Input: part model. Units: mm. Frame: model coordinates. A direction names the side the tool comes from. Coordinates: 2 decimals unless noted, no trailing zeros. Order: outer loops, then holes, each group sorted by start corner. A loop starts at its lowest first (then second) coordinate and runs counter-clockwise, first axis right, second up. Notation, with made-up numbers: (-39, 64) -> (-20, 64) arc R26 cw to (-20, 97) -> close; hole circle Ø4 at (7.5, 7.5). An arc over 180 degrees is marked (long way). Use one line per item in the form item = value. Start each with the question number.
1) Pin query (flat end, axial travel): pin 1 (4 mm diameter, centred on x = 17.5, y = -8, fed in from +Z); pin 2 (0.9 mm diameter, centred on x = 63, y = 21.5, fed in from +Z); pin 3 (1 mm diameter, centred on x = 22, y = 17.5, fed in from +Z); pin 4 (2.5 mm diameter, centred on x = 68.6, z = 64, fed in from +Y). Return the tip coordinate at first contact, or that it passes through.
2) Draft query along Z for faces 1 (the flat face through (-7.6, 16.25, 9.93)), 2 (the cylindrical face through (-11.53, 21.52, -17.5)), 3 (the cylindrical face through (28.83, 22.24, 65.004)). Return one class per face: pulls with the +Z half, pulls with the -Z half, needs draft (parallel to the pull), parting line crosses it, or undercut.
3) Section query C-C on z = 29. Output: boundary loops of the cut face in (x, y).
4) Ray query, line 1 along X through (y, z) = (21.65, 64); line 2 along Z through (x, y) = (68.6, 22.3); line 3 along X through (y, z) = (22, -16). Return the intervals inside material, ascending.
5) Access query for faces 4 (the flat face through (19, -7, 4)), 5 (the flat face through (18, -3.5, 3)), 6 (the flat face through (0, 22, -9)), 7 (the flat face through (64, 21, 74)). Directions: +Z, -Z, +X, -X, +Y, -Y. A direction counts if a zero-diameter tool reaches every point of the face in a straight line with its end or side. Return the directions, or none.
6) Section query A-A on z = -4. Output: boundary loops of the cut face in (x, y).
7) Section query B-B on y = -8. Count the separate pieces of the cut face and the enclosed holes in it, then the cut area to 3 significant figures.
from build123d import *

# Parameters (mm, degrees)
SKETCH_1_W               = 57
SKETCH_1_H               = 23
EXTRUDE_1_DEPTH          = 80
SKETCH_2_W               = 55
SKETCH_2_H               = 20
CUT_EXTRUDE_1_DEPTH      = 75
SKETCH_3_W               = 6
SKETCH_3_H               = 6
EXTRUDE_2_DEPTH          = 6
SKETCH_4_W               = 6
SKETCH_4_H               = 6.5
SKETCH_4_R               = 1.5
EXTRUDE_3_DEPTH          = 3
MIRROR_2_COPY_1_SKETCH_W = 6
MIRROR_2_COPY_1_SKETCH_H = 6.5
MIRROR_2_COPY_1_SKETCH_R = 1.5
MIRROR_2_COPY_1_DEPTH    = 3
CUT_EXTRUDE_3_DEPTH      = 104.624321469
CUT_EXTRUDE_3_DEPTH_BACK = 25
SKETCH_6_W               = 38
SKETCH_6_H               = 3
SKETCH_6_W_2             = 20
EXTRUDE_4_DEPTH          = 15
SKETCH_8_R               = 1.5
CUT_EXTRUDE_4_DEPTH      = 113.57441983
EXTRUDE_5_DEPTH          = 5


with BuildPart() as part:
    # 草图1 → 凸台-拉伸1 (new body)
    with BuildSketch(Plane.XY):
        with Locations((28.5, 11.5)):
            Rectangle(SKETCH_1_W, SKETCH_1_H)
    extrude(amount=EXTRUDE_1_DEPTH)

    # 草图2 → 切除-拉伸1 (cut)
    with BuildSketch(Plane.XY.offset(80)):
        with Locations((28.5, 11.5)):
            Rectangle(SKETCH_2_W, SKETCH_2_H)
    extrude(amount=-CUT_EXTRUDE_1_DEPTH, mode=Mode.SUBTRACT)

    # 草图3 → 凸台-拉伸2 (add)
    with BuildSketch(Plane.XZ):
        with Locations((17.5, 62)):
            Rectangle(SKETCH_3_W, SKETCH_3_H)
        with Locations((17.5, 7)):
            Rectangle(SKETCH_3_W, SKETCH_3_H)
        with Locations((39.5, 7)):
            Rectangle(SKETCH_3_W, SKETCH_3_H)
        with Locations((39.5, 62)):
            Rectangle(SKETCH_3_W, SKETCH_3_H)
    extrude(amount=EXTRUDE_2_DEPTH)

    # 草图4 → 凸台-拉伸3 (add)
    with BuildSketch(Plane.XY.offset(65)):
        with Locations((39.5, -6.75)):
            Rectangle(SKETCH_4_W, SKETCH_4_H)
        with Locations((39.5, -8)):
            Circle(SKETCH_4_R, mode=Mode.SUBTRACT)
    extrude_3 = extrude(amount=EXTRUDE_3_DEPTH)

    # 镜向1: 凸台-拉伸3 across plane
    add(extrude_3.mirror(Plane.XY.offset(34.5)))

    # 镜向2: 凸台-拉伸3 across plane
    add(extrude_3.mirror(Plane.ZY.offset(-28.5)))

    # 镜向2 copy 1 sketch → 镜向2 copy 1 (add)
    with BuildSketch(Plane(origin=(57, 0, 4), x_dir=(-1, 0, 0), z_dir=(0, 0, -1))):
        with Locations((39.5, -6.75)):
            Rectangle(MIRROR_2_COPY_1_SKETCH_W, MIRROR_2_COPY_1_SKETCH_H)
        with Locations((39.5, -8)):
            Circle(MIRROR_2_COPY_1_SKETCH_R, mode=Mode.SUBTRACT)
    extrude(amount=MIRROR_2_COPY_1_DEPTH)

    # 草图5 → 切除-拉伸3 (cut, two sides: drawn at the far end of the back side and taken through both)
    with BuildSketch(Plane(origin=(0, 23, 0), x_dir=(1, 0, 0), z_dir=(0, 1, 0)).offset(-CUT_EXTRUDE_3_DEPTH_BACK)):
        with BuildLine():
            Line((43.5, -272.123584415), (43.5, -80))
            ThreePointArc((43.5, -80), (28.5, -65), (13.5, -80))
            Line((13.5, -80), (13.5, -272.123584415))
            Line((13.5, -272.123584415), (13.5, -656.370753244))
            Line((13.5, -656.370753244), (43.5, -656.370753244))
            Line((43.5, -656.370753244), (43.5, -272.123584415))
        make_face()
    extrude(amount=CUT_EXTRUDE_3_DEPTH + CUT_EXTRUDE_3_DEPTH_BACK, mode=Mode.SUBTRACT)

    # 草图6 → 凸台-拉伸4 (add)
    with BuildSketch(Plane.ZY):
        with Locations((1, 21.5)):
            Rectangle(SKETCH_6_W, SKETCH_6_H)
        with Locations((64, 21.5)):
            Rectangle(SKETCH_6_W_2, SKETCH_6_H)
    extrude_4 = extrude(amount=EXTRUDE_4_DEPTH)

    # 镜向3: 凸台-拉伸4 across plane
    add(extrude_4.mirror(Plane.ZY.offset(-28.5)))

    # 草图8 → 切除-拉伸4 (cut, through all)
    with BuildSketch(Plane(origin=(0, 23, 0), x_dir=(1, 0, 0), z_dir=(0, 1, 0))):
        with Locations(Location((-11.6, 16, 0), (0, 0, 270))):
            Circle(SKETCH_8_R)
        with Locations(Location((68.6, 16, 0), (0, 0, 90))):
            Circle(SKETCH_8_R)
        with Locations(Location((-11.6, -64, 0), (0, 0, 270))):
            Circle(SKETCH_8_R)
        with Locations(Location((68.6, -64, 0), (0, 0, 270))):
            Circle(SKETCH_8_R)
    extrude(amount=-CUT_EXTRUDE_4_DEPTH, mode=Mode.SUBTRACT)

    # 草图12 → 凸台-拉伸5 (add, symmetric)
    with BuildSketch(Plane(origin=(0, 0, 10), x_dir=(-1, 0, 0), z_dir=(0, 0, -1))):
        Polygon((15, 20), (0, 12.4), (0, 14), (11.842105263, 20), align=None)
    extrude_5 = extrude(amount=EXTRUDE_5_DEPTH, both=True)

    # 镜向4: 凸台-拉伸5 across plane
    add(extrude_5.mirror(Plane.ZY.offset(-28.5)))


solid = part.part
Answers below:
q1.pin_1 = 68
q1.pin_2 = 74
q1.pin_3 = 5
q1.pin_4 = through
q2.face_1 = needs draft
q2.face_2 = undercut
q2.face_3 = pulls with the +Z half
q3.outline = (0, 0) -> (57, 0) -> (57, 23) -> (0, 23) -> close; hole (1, 1.5) -> (56, 1.5) -> (56, 21.5) -> (1, 21.5) -> close
q4.line_1 = -15 to -13.1, -10.1 to 67.1, 70.1 to 72
q4.line_2 = -18 to -17.5, -14.5 to 20, 54 to 62.5, 65.5 to 74
q4.line_3 = -15 to -13.1, -10.1 to 0, 57 to 67.1, 70.1 to 72
q5.face_4 = +X, -X, -Y
q5.face_5 = -Z, +X, -X
q5.face_6 = -Z, +Y, -Y
q5.face_7 = +Z, +X, +Y, -Y
q6.outline = (-15, 20) -> (0, 20) -> (0, 23) -> (-15, 23) -> close; (57, 20) -> (72, 20) -> (72, 23) -> (57, 23) -> close
q7.separate_pieces = 8
q7.enclosed_holes = 0
q7.area = 36.0 mm^2
